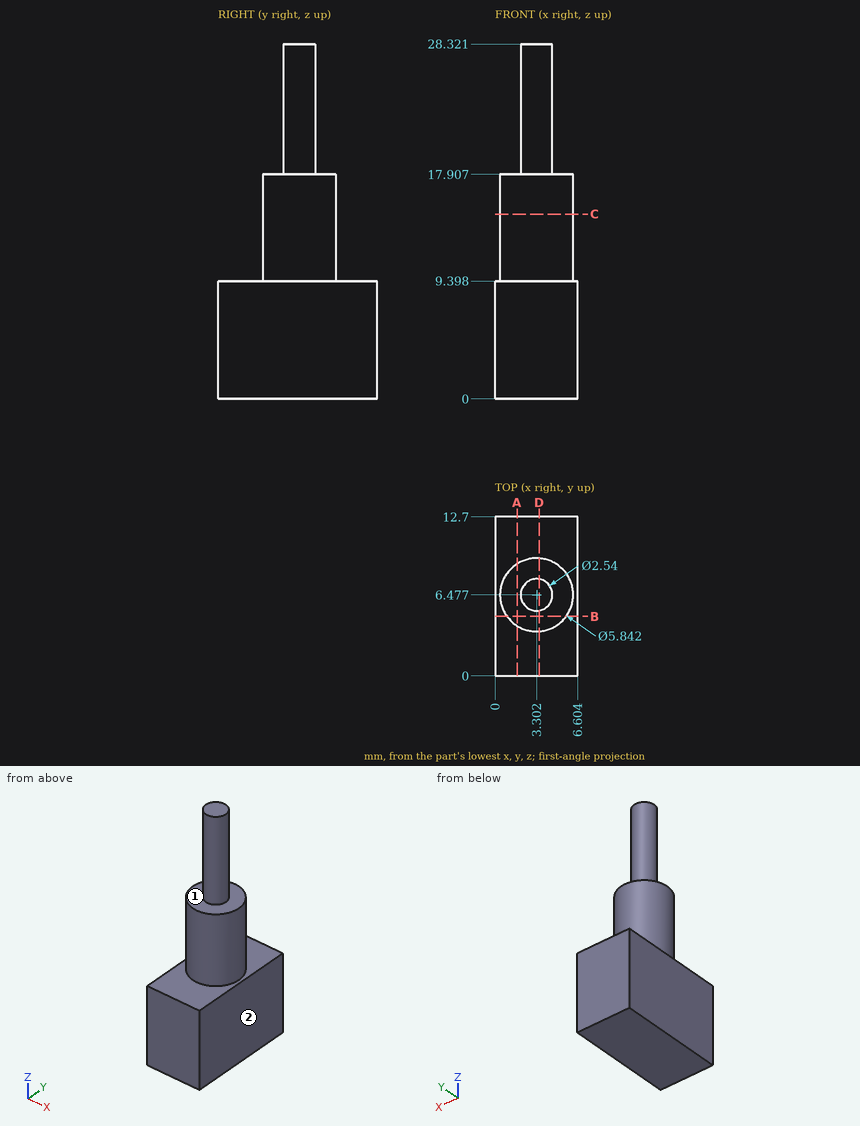
Can you work these out from the drawing? Everything is in mm from the part's minimum corner. A direction names the side the tool comes from. Coordinates: 2 decimals unless noted, no trailing zeros. Order: outer loops, then holes, each group sorted by start corner. A loop starts at its lowest first (then second) coordinate and runs counter-clockwise, first axis right, second up. Notation, with made-up numbers: (70, 36) -> (107, 36) arc R34 ccw to (107, 72) -> close; hole circle Ø5 at (-16, -6). An arc over 180 degrees is marked (long way). Use one line per item in the form item = value.
Q1. I need wall thicknesses on L1, parallel to Z at x = 1.5, y = 2.75; L2, parallel to X at y = 6.5, z = 17; L3, parallel to Z at x = 2, y = 6.5. Which ranges of each line are inside material? Lowest first, please.
From the geometry:
L1 = 0 to 9.4
L2 = 0.38 to 6.22
L3 = 0 to 17.91
Q2. Which directions (+Z, -Z, +X, -X, +Y, -Y) give clear straight access to the entire face, cutting with the end or side of a thin tool? Please do the marked faces 1 and 2.
From the geometry:
face_1 = +Z
face_2 = +Z, -Z, +X, +Y, -Y
Q3. Will these pins go through, and if not, where does the flat tip stop? P1, Ø4, axis at y = 10, z = 7, coming from the -X side; P2, Ø1.5, axis at x = 3.5, z = 13, coming from the -Y side; P3, Ø3, axis at x = 2.5, z = 25.5, coming from the -Y side; P4, Ø6, axis at y = 4, z = 13, coming from the -X side.
From the geometry:
P1 = 0
P2 = 3.56
P3 = 5.21
P4 = 0.38
Q4. Imagine slicing it at C-C, the plane z = 14.75. List the corners of the cut face in (x, y) for me, then the cut area to 3 significant figures.
From the geometry:
outline = circle Ø5.84 at (3.3, 6.48)
area = 26.8 mm²
Q5. Imagine slicing it at A-A, the plane x = 1.75. List the corners of the cut face in (y, z) for me.
From the geometry:
outline = (0, 0) -> (12.7, 0) -> (12.7, 9.4) -> (8.95, 9.4) -> (8.95, 17.91) -> (4, 17.91) -> (4, 9.4) -> (0, 9.4) -> close
Q6. Imagine slicing it at B-B, the plane y = 4.75. List the corners of the cut face in (x, z) for me, then the cut area to 3 significant figures.
From the geometry:
outline = (0, 0) -> (6.6, 0) -> (6.6, 9.4) -> (5.66, 9.4) -> (5.66, 17.91) -> (0.95, 17.91) -> (0.95, 9.4) -> (0, 9.4) -> close
area = 102 mm²
Q7. Imagine slicing it at D-D, the plane x = 3.5. List the corners of the cut face in (y, z) for me.
From the geometry:
outline = (0, 0) -> (12.7, 0) -> (12.7, 9.4) -> (9.39, 9.4) -> (9.39, 17.91) -> (7.73, 17.91) -> (7.73, 28.32) -> (5.22, 28.32) -> (5.22, 17.91) -> (3.56, 17.91) -> (3.56, 9.4) -> (0, 9.4) -> close
